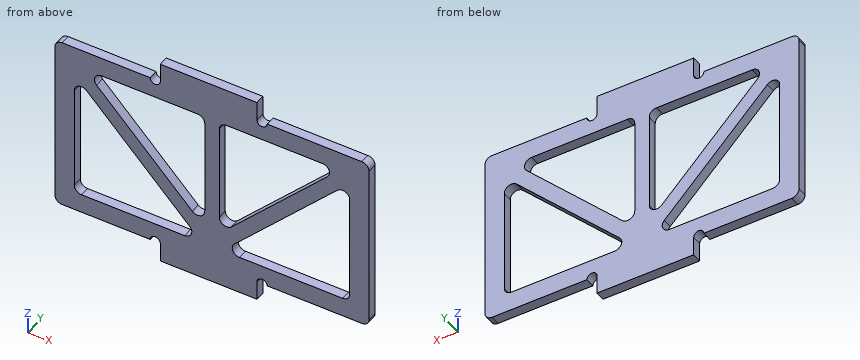
from build123d import *

# Parameters (mm, degrees)
SKETCH_1_W          = 65
SKETCH_1_H          = 37
EXTRUDE_1_DEPTH     = 2
SKETCH_2_W          = 20
SKETCH_2_H          = 2
EXTRUDE_2_DEPTH     = 4
SKETCH_3_R          = 1.05
CUT_EXTRUDE_1_DEPTH = 4
CUT_EXTRUDE_2_DEPTH = 10
FILLET_1_R          = 1.5


with BuildPart() as part:
    # 草图1 → 凸台-拉伸1 (new body)
    with BuildSketch(Plane(origin=(0, 0, 0), x_dir=(1, 0, 0), z_dir=(0, 1, 0))):
        Rectangle(SKETCH_1_W, SKETCH_1_H)
    extrude(amount=EXTRUDE_1_DEPTH)

    # 草图2 → 凸台-拉伸2 (add)
    with BuildSketch(Plane(origin=(0, 0, -18.5), x_dir=(-1, 0, 0), z_dir=(0, 0, -1))):
        with Locations((0.7, 1)):
            Rectangle(SKETCH_2_W, SKETCH_2_H)
    extrude_2 = extrude(amount=EXTRUDE_2_DEPTH)

    # 镜向1: 凸台-拉伸2 across plane
    add(extrude_2.mirror(Plane.XY))

    # 草图3 → 切除-拉伸1 (cut)
    with BuildSketch(Plane(origin=(0, 2, 0), x_dir=(1, 0, 0), z_dir=(0, 1, 0))):
        with Locations((10.35, -18.5)):
            Circle(SKETCH_3_R)
        with Locations((-11.75, -18.5)):
            Circle(SKETCH_3_R)
        with Locations((-11.75, 18.5)):
            Circle(SKETCH_3_R)
        with Locations((10.35, 18.5)):
            Circle(SKETCH_3_R)
    extrude(amount=-CUT_EXTRUDE_1_DEPTH, mode=Mode.SUBTRACT)

    # 草图4 → 切除-拉伸2 (cut)
    with BuildSketch(Plane(origin=(0, 2, 0), x_dir=(1, 0, 0), z_dir=(0, 1, 0))):
        Polygon((-28.5, 14.5), (-28.5, -12.35999068), (-2.103112607, 14.5), align=None)
        Polygon((-26.396887393, -14.5), (-1.5, -14.5), (-1.5, 10.833674891), align=None)
        Polygon((1.5, 10.833674891), (1.5, -14.5), (26.396887393, -14.5), align=None)
        Polygon((2.103112607, 14.5), (28.5, -12.35999068), (28.5, 14.5), align=None)
    extrude(amount=-CUT_EXTRUDE_2_DEPTH, mode=Mode.SUBTRACT)

    # 圆角1
    fillet_1_edges = [part.edges().sort_by_distance(p)[0] for p in [
        (2.103112607, 1, -14.5),
        (28.5, 1, -14.5),
        (28.5, 1, 12.35999068),
        (-2.103112607, 1, -14.5),
        (-28.5, 1, 12.35999068),
        (-28.5, 1, -14.5),
        (32.5, 1, 18.5),
        (-32.5, 1, 18.5),
        (-32.5, 1, -18.5),
        (32.5, 1, -18.5),
        (-1.5, 1, -10.833674891),
        (-1.5, 1, 14.5),
        (-26.396887393, 1, 14.5),
        (1.5, 1, -10.833674891),
        (26.396887393, 1, 14.5),
        (1.5, 1, 14.5),
    ]]
    fillet(fillet_1_edges, radius=FILLET_1_R)


solid = part.part
Source: CAD feature listing. Evaluate the final solid. Frame: model axes, mm. Round coordinates to 2 decimals unless told otherwise and drop trailing zeros. Write each loop counter-clockwise with the first axis right and the second up, starting at its lowest first coordinate (ties: lowest second). Pieces come first, ordered by that corner, then holes. Notation, with made-up numbers: M -8.75,-29.5 L -1.75,-29.5 A23 ccw -1.75,-9.5 Z; hole C 88.25,5 d2. An arc over 180 degrees is marked long. One line per item, written item: value. Start each with the question number.
Item 1: Section query D-D (y = 0.35). State how many separate pieces and enclosed holes the cut face has, plus the area to 3 significant figures.
Item 2: Section query B-B (z = 7.5). Return the cut outline in (x, y), plus the area to 3 significant figures.
Item 3: Ray query, L1, parallel to X at y = 0.25, z = 13; L2, parallel to Z at x = 19, y = 1.15; L3, parallel to X at y = 1, z = -2. Return the intervals inside material, ascending. Write a range as from..to.
Item 4: Pin query (flat end, axial travel): pin 1 (0.6 mm diameter, centred on x = 13.5, y = 1, fed in from +Z); pin 2 (0.6 mm diameter, centred on y = 1, z = -20, fed in from -X); pin 3 (0.6 mm diameter, centred on x = 22.5, y = 1, fed in from -Z). Return the tip coordinate at first contact, or that it passes through.
Item 5: Section query A-A (x = 15.5). Return the cut outline in (y, z).
Item 6: Section query C-C (x = -25). Return the cut outline in (y, z).
Result set:
1. separate pieces: 1
1. enclosed holes: 4
1. area: 1,240 mm²
2. outline: M -32.5,0 L -28.5,0 L -28.5,2 L -32.5,2 Z; M -23.72,0 L -19.52,0 L -19.52,2 L -23.72,2 Z; M -1.5,0 L 1.5,0 L 1.5,2 L -1.5,2 Z; M 19.52,0 L 23.72,0 L 23.72,2 L 19.52,2 Z; M 28.5,0 L 32.5,0 L 32.5,2 L 28.5,2 Z
2. area: 38.8 mm²
3. L1: x = -32.5..-24.32, -1.5..1.5, 24.32..32.5
3. L2: z = -18.5..-14.5, 2.69..6.97, 14.5..18.5
3. L3: x = -32.5..-28.5, -14.39..-10.18, -1.5..1.5, 10.18..14.39, 28.5..32.5
4. pin 1: stops at z = 18.5
4. pin 2: stops at x = -10.7
4. pin 3: stops at z = -18.5
5. outline: M 0,-18.5 L 2,-18.5 L 2,-14.5 L 0,-14.5 Z; M 0,-0.87 L 2,-0.87 L 2,3.41 L 0,3.41 Z; M 0,14.5 L 2,14.5 L 2,18.5 L 0,18.5 Z
6. outline: M 0,-18.5 L 2,-18.5 L 2,-14.5 L 0,-14.5 Z; M 0,8.8 L 2,8.8 L 2,18.5 L 0,18.5 Z
